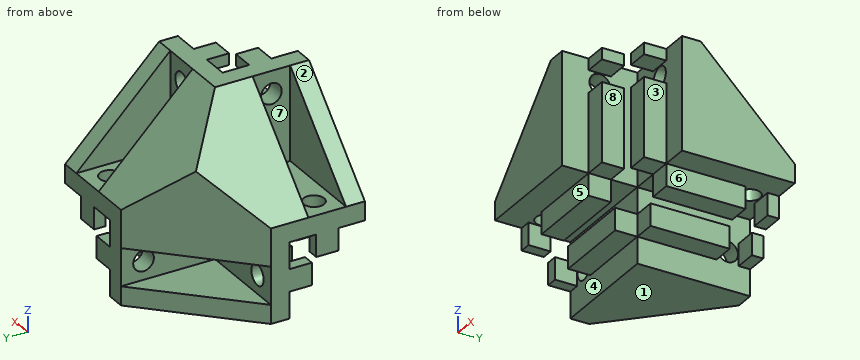
```python
from build123d import *

# Parameters (mm, degrees)
F0_W      = 20
F0_H      = 30
F0_W_2    = 30
F0_H_2    = 20
F1_DEPTH  = 50
F2_DEPTH  = 20
F3_SIZE   = 25
F6_DEPTH  = 10
F9_DEPTH  = 10
F12_DEPTH = 10
F13_R     = 2.75
F14_DEPTH = 5
F15_R     = 2.75
F16_DEPTH = 5
F17_R     = 2.75
F18_DEPTH = 5
F19_R     = 2.75
F20_DEPTH = 5
F21_R     = 2.75
F22_DEPTH = 5
F23_R     = 2.75
F24_DEPTH = 5
F25_W     = 5.9
F25_H     = 21.05
F25_H_2   = 3.05
F26_DEPTH = 5.9
F27_W     = 5.9
F27_H     = 3.04
F27_H_2   = 21.06
F28_DEPTH = 5.9
F29_W     = 26.96
F29_H     = 5.9
F29_W_2   = 3.04
F30_DEPTH = 5.9
F31_W     = 5.9
F31_H     = 26.94
F31_H_2   = 3.06
F32_DEPTH = 5.9
F33_W     = 21.06
F33_H     = 5.9
F33_W_2   = 3.04
F34_DEPTH = 5.9
F35_W     = 26.95
F35_H     = 5.9
F35_W_2   = 3.05
F36_DEPTH = 5.9
F37_W     = 5.9
F37_H     = 5.9
F38_DEPTH = 5.9
F39_W     = 5.9
F39_H     = 5.9
F40_DEPTH = 5.9
F41_W     = 5.9
F41_H     = 5.9
F42_DEPTH = 5.9


with BuildPart() as f1:
    # F0 (on Top) → F1 (new body)
    with BuildSketch(Plane.XY):
        with Locations((15, 10)):
            Rectangle(F0_W, F0_H)
        Polygon((5, -5), (5, 25), (0, 25), (-25, 0), (-25, -5), align=None)
        with Locations((-10, -15)):
            Rectangle(F0_W_2, F0_H_2)
    extrude(amount=F1_DEPTH)

    # F0 (on Top) → F2 (cut)
    with BuildSketch(Plane.XY):
        with Locations((-10, -15)):
            Rectangle(F0_W_2, F0_H_2)
        with Locations((15, 10)):
            Rectangle(F0_W, F0_H)
    extrude(amount=F2_DEPTH, mode=Mode.SUBTRACT)

    # F3 (call 1 of 2: OpenCascade refuses the feature's edges together)
    f3_edges = [f1.edges().sort_by_distance(p)[0] for p in [
        (12.5, 25, 50),
    ]]
    chamfer(f3_edges, length=F3_SIZE)

    # F3#2 (call 2 of 2)
    f3_2_edges = [f1.edges().sort_by_distance(p)[0] for p in [
        (-25, -12.5, 50),
    ]]
    chamfer(f3_2_edges, length=F3_SIZE)

    # F5 (on offset) → F6 (cut)
    with BuildSketch(Plane.YZ.offset(20)):
        Polygon((0, 25), (25, 25), (0, 50), align=None)
    extrude(amount=-F6_DEPTH, mode=Mode.SUBTRACT)

    # F8 (on offset) → F9 (cut)
    with BuildSketch(Plane.XZ.offset(20)):
        Polygon((0, 25), (0, 50), (-25, 25), align=None)
    extrude(amount=-F9_DEPTH, mode=Mode.SUBTRACT)

    # F11 (on offset) → F12 (cut)
    with BuildSketch(Plane.XY.offset(5)):
        Polygon((0, 0), (0, 25), (-25, 0), align=None)
    extrude(amount=F12_DEPTH, mode=Mode.SUBTRACT)

    # F13 (on face) → F14 (cut)
    with BuildSketch(Plane(origin=(0, 0, 0), x_dir=(0, -1, 0), z_dir=(-1, 0, 0))):
        with Locations((15, 44)):
            Circle(F13_R)
    extrude(amount=-F14_DEPTH, mode=Mode.SUBTRACT)

    # F15 (on face) → F16 (cut)
    with BuildSketch(Plane.XY.offset(25)):
        with Locations((-19, -15)):
            Circle(F15_R)
    extrude(amount=-F16_DEPTH, mode=Mode.SUBTRACT)

    # F17 (on face) → F18 (cut)
    with BuildSketch(Plane(origin=(0, 0, 0), x_dir=(-1, 0, 0), z_dir=(0, 1, 0))):
        with Locations((19, 10)):
            Circle(F17_R)
    extrude(amount=-F18_DEPTH, mode=Mode.SUBTRACT)

    # F19 (on face) → F20 (cut)
    with BuildSketch(Plane(origin=(0, 0, 0), x_dir=(0, -1, 0), z_dir=(-1, 0, 0))):
        with Locations((-19, 10)):
            Circle(F19_R)
    extrude(amount=-F20_DEPTH, mode=Mode.SUBTRACT)

    # F21 (on face) → F22 (cut)
    with BuildSketch(Plane.XY.offset(25)):
        with Locations((15, 19)):
            Circle(F21_R)
    extrude(amount=-F22_DEPTH, mode=Mode.SUBTRACT)

    # F23 (on face) → F24 (cut)
    with BuildSketch(Plane(origin=(0, 0, 0), x_dir=(-1, 0, 0), z_dir=(0, 1, 0))):
        with Locations((-15, 44)):
            Circle(F23_R)
    extrude(amount=-F24_DEPTH, mode=Mode.SUBTRACT)

    # F25 (on face) → F26 (join)
    with BuildSketch(Plane.XZ.offset(5)):
        with Locations((15, 30.525)):
            Rectangle(F25_W, F25_H)
        with Locations((15, 48.475)):
            Rectangle(F25_W, F25_H_2)
    extrude(amount=F26_DEPTH)

    # F27 (on face) → F28 (join)
    with BuildSketch(Plane.YZ.offset(5)):
        with Locations((-15, 48.48)):
            Rectangle(F27_W, F27_H)
        with Locations((-15, 30.53)):
            Rectangle(F27_W, F27_H_2)
    extrude(amount=F28_DEPTH)

    # F29 (on face) → F30 (join)
    with BuildSketch(Plane(origin=(0, 0, 20), x_dir=(1, 0, 0), z_dir=(0, 0, -1))):
        with Locations((-2.58, 15)):
            Rectangle(F29_W, F29_H)
        with Locations((-23.48, 15)):
            Rectangle(F29_W_2, F29_H)
    extrude(amount=F30_DEPTH)

    # F31 (on face) → F32 (join)
    with BuildSketch(Plane(origin=(0, 0, 20), x_dir=(1, 0, 0), z_dir=(0, 0, -1))):
        with Locations((15, -2.57)):
            Rectangle(F31_W, F31_H)
        with Locations((15, -23.47)):
            Rectangle(F31_W, F31_H_2)
    extrude(amount=F32_DEPTH)

    # F33 (on face) → F34 (join)
    with BuildSketch(Plane.YZ.offset(5)):
        with Locations((5.53, 10)):
            Rectangle(F33_W, F33_H)
        with Locations((23.48, 10)):
            Rectangle(F33_W_2, F33_H)
    extrude(amount=F34_DEPTH)

    # F35 (on face) → F36 (join)
    with BuildSketch(Plane.XZ.offset(5)):
        with Locations((-2.575, 10)):
            Rectangle(F35_W, F35_H)
        with Locations((-23.475, 10)):
            Rectangle(F35_W_2, F35_H)
    extrude(amount=F36_DEPTH)

    # F37 (on face) → F38 (cut)
    with BuildSketch(Plane(origin=(0, 0, 7.05), x_dir=(1, 0, 0), z_dir=(0, 0, -1))):
        with Locations((7.95, 7.95)):
            Rectangle(F37_W, F37_H)
    extrude(amount=-F38_DEPTH, mode=Mode.SUBTRACT)

    # F39 (on face) → F40 (cut)
    with BuildSketch(Plane(origin=(0, 0, 14.1), x_dir=(1, 0, 0), z_dir=(0, 0, -1))):
        with Locations((7.95, 15)):
            Rectangle(F39_W, F39_H)
    extrude(amount=-F40_DEPTH, mode=Mode.SUBTRACT)

    # F41 (on face) → F42 (cut)
    with BuildSketch(Plane(origin=(0, 0, 14.1), x_dir=(1, 0, 0), z_dir=(0, 0, -1))):
        with Locations((15, 7.95)):
            Rectangle(F41_W, F41_H)
    extrude(amount=-F42_DEPTH, mode=Mode.SUBTRACT)


solid = f1.part
```
Here's how the part is built. I have some questions about the finished solid (model axes, mm). Face numbers are marked on the shaded views. A direction names the side the tool comes from. Coordinates: 2 decimals unless noted, no trailing zeros. Loops run counter-clockwise (first coordinate to the right, second up) from the corner with the lowest first, then second, coordinate; pieces in that order, holes last. Notation, with made-up numbers: (-2.5, -13.5) - (43.5, -13.5) arc R12 cw to (43.5, -7.5) - close; hole circle Ø4 at (80.5, 9.5). An arc over 180 degrees is marked (long way). Return JSON: item names as keys, results as strings. Group by question number.
Item 1: If we section it at C-C on x = -3.5: Write out the boundary of the cut face in (y, z), and give its area (3 significant figures).
Item 2: If we section it at A-A on y = -15: Write out the boundary of the cut face in (x, z).
Item 3: I need wall thicknesses on line 1 (X direction, y = -15, z = 18); line 2 (X direction, y = 15, z = 30); line 3 (Z direction, x = 1.3, y = -15). Which ranges of each line are inside material? Lowest first, please. Write a range as from..to.
Item 4: We'd pull the mould along Z, two halves only. Please class the marked faces 1, 2, 3 and 4: +Z half, -Z half, draft (parallel to the pull), parting line (faces both ways), or undercut.
Item 5: Will these pins go through, and if not, where does the flat tip stop? P1, Ø3, axis at x = -7.5, z = 15.5, coming from the +Y side; P2, Ø1.8, axis at x = -2.5, z = 16.5, coming from the -Y side; P3, Ø16, axis at x = -11, y = -16, coming from the -Z side.
Item 6: If we section it at B-B on z = 44: Write out the boundary of the cut face in (x, y), and give its area (3 significant figures).
Item 7: On a 3-axis mill with a long thin cutter (end or side, diameter ignored), from which of +Z, -Z, +X, -X, +Y, -Y can I reach the whole of each face in a straight line? I mean the marked faces 5, 6, 7 and 8. Say none if no direction works.
Item 8: If we section it at D-D on y = -1.5: Write out the boundary of the cut face in (x, z), and give its area (3 significant figures).
Calculated:
{
 "1": {"outline": "(-25, 20) - (-17.95, 20) - (-17.95, 14.1) - (-12.05, 14.1) - (-12.05, 20) - (-5, 20) - (-5, 12.95) - (-10.9, 12.95) - (-10.9, 7.05) - (-5, 7.05) - (-5, 0) - (21.5, 0) - (21.5, 5) - (0, 5) - (0, 15) - (21.5, 15) - (21.5, 28.5) - (3.5, 46.5) - (-10, 46.5) - (-10, 25) - (-20, 25) - (-20, 46.5) - (-25, 46.5) - close", "area": "1,240 mm^2"},
 "2": {"outline": "(-25, 14.1) - (-21.96, 14.1) - (-21.96, 20) - (-21.75, 20) - (-21.75, 25) - (-25, 25) - close; (-16.25, 20) - (-16.06, 20) - (-16.06, 14.1) - (5, 14.1) - (5, 20) - (10.9, 20) - (10.9, 41.06) - (5, 41.06) - (5, 41.25) - (0, 41.25) - (0, 25) - (-16.25, 25) - close; (0, 46.75) - (5, 46.75) - (5, 46.96) - (10.9, 46.96) - (10.9, 50) - (0, 50) - close"},
 "3": {"line 1": "x = -25..-21.96, -16.06..5", "line 2": "x = -10..10, 20..25", "line 3": "z = 14.1..41.25, 46.75..50"},
 "4": {"face 1": "-Z half", "face 2": "+Z half", "face 3": "draft", "face 4": "undercut"},
 "5": {"P1": "stops at y = 19", "P2": "stops at y = -17.95", "P3": "stops at z = 7.05"},
 "6": {"outline": "(-6, -25) - (5, -25) - (5, -17.75) - (0, -17.75) - (0, -20) - (-6, -20) - close; (-6, -10) - (0, -10) - (0, -12.25) - (5, -12.25) - (5, -5) - (12.25, -5) - (12.25, 0) - (10, 0) - (10, 6) - (-6, 6) - close; (17.75, -5) - (25, -5) - (25, 6) - (20, 6) - (20, 0) - (17.75, 0) - close", "area": "386 mm^2"},
 "7": {"face 5": "-Z, +X, -X, -Y", "face 6": "-Z, +X, +Y, -Y", "face 7": "+Z, -X", "face 8": "+Z, -Z, +X, -Y"},
 "8": {"outline": "(-25, 0) - (5, 0) - (5, 7.05) - (10.9, 7.05) - (10.9, 12.95) - (5, 12.95) - (5, 20) - (12.05, 20) - (12.05, 14.1) - (17.95, 14.1) - (17.95, 20) - (25, 20) - (25, 50) - (0, 50) - (-25, 25) - close; hole circle Ø5.5 at (-19, 10); hole circle Ø5.5 at (15, 44)", "area": "1,810 mm^2"}
}
